Print and shaded views of the part. All mm, measured from the part's lowest x, y and z. A direction names the side the tool comes from. Round coordinates to 2 decimals unless told otherwise and drop trailing zeros. Write each loop counter-clockwise with the first axis right and the second up, starting at its lowest first coordinate (ties: lowest second). Pieces come first, ordered by that corner, then holes. Notation, with made-up numbers: M 69.5,-22.75 L 122.5,-22.75 A11 cw 122.5,-11.75 Z; hole C 26,-10 d8. An arc over 180 degrees is marked long. Write item = value, one per line.
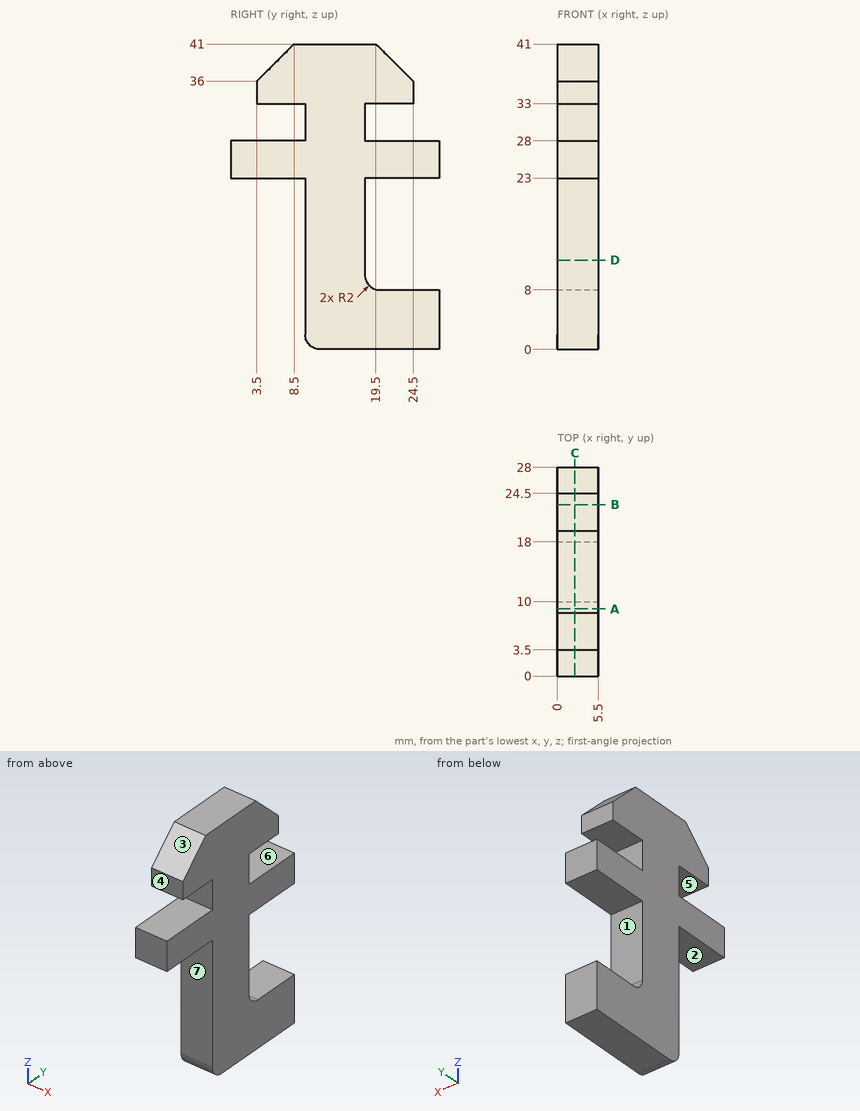
1. Mould opens along Z. For the marked faces 1, 2 and 3 say: pulls with the +Z half, pulls with the -Z half, needs draft (parallel to the pull), parting line crosses it, or undercut.
Responses:
face_1 = undercut
face_2 = pulls with the -Z half
face_3 = pulls with the +Z half
2. Band-saw the part on B-B (y = 23). List the corners of the cut face in (x, z).
Responses:
outline = M 0,0 L 5.5,0 L 5.5,8 L 0,8 Z; M 0,23 L 5.5,23 L 5.5,28 L 0,28 Z; M 0,33 L 5.5,33 L 5.5,37.5 L 0,37.5 Z
3. Band-saw the part on D-D (z = 12). List the corners of the cut face in (x, y).
Responses:
outline = M 0,10 L 5.5,10 L 5.5,18 L 0,18 Z
4. Probe probe 1 along Z at (x, y) = (3.8, 20.75); probe 2 along Z at (x, y) = (4.4, 25.5); probe 3 along Z at (x, y) = (4.6, 20.5). List the from-to ranges inside material, lowest first.
Responses:
probe_1 = 0 to 8, 23 to 28, 33 to 39.75
probe_2 = 0 to 8, 23 to 28
probe_3 = 0 to 8, 23 to 28, 33 to 40
5. Tool access for the marked faces 4, 5, 6 and 7: list every direction of +Z, -Z, +X, -X, +Y, -Y with a clear straight run to the whole face (end or side of a thin tool).
Responses:
face_4 = +Z, +X, -X, -Y
face_5 = +X, -X, -Y
face_6 = +X, -X, +Y
face_7 = -Z, +X, -X, -Y
6. Band-saw the part on C-C (x = 2.35). List the corners of the cut face in (y, z), plus the area to 3 significant figures.
Responses:
outline = M 0,23 L 10,23 L 10,2 A2 ccw 12,0 L 28,0 L 28,8 L 20,8 A2 cw 18,10 L 18,23 L 28,23 L 28,28 L 18,28 L 18,33 L 24.5,33 L 24.5,36 L 19.5,41 L 8.5,41 L 3.5,36 L 3.5,33 L 10,33 L 10,28 L 0,28 Z
area = 587 mm²
7. Flat gauge pins, fed straight in: pin 1 (1 mm diameter, centred on x = 2.5, z = 18, fed in from +Y); pin 2 (3 mm diameter, centred on x = 4, y = 24, fed in from +Z); pin 3 (1.6 mm diameter, centred on x = 2, y = 6, fed in from +Z). Where does each tip first touch, or does it go through?
Responses:
pin_1 = 18
pin_2 = 38
pin_3 = 39.3
8. Band-saw the part on A-A (y = 9). List the corners of the cut face in (x, z).
Responses:
outline = M 0,23 L 5.5,23 L 5.5,28 L 0,28 Z; M 0,33 L 5.5,33 L 5.5,41 L 0,41 Z
